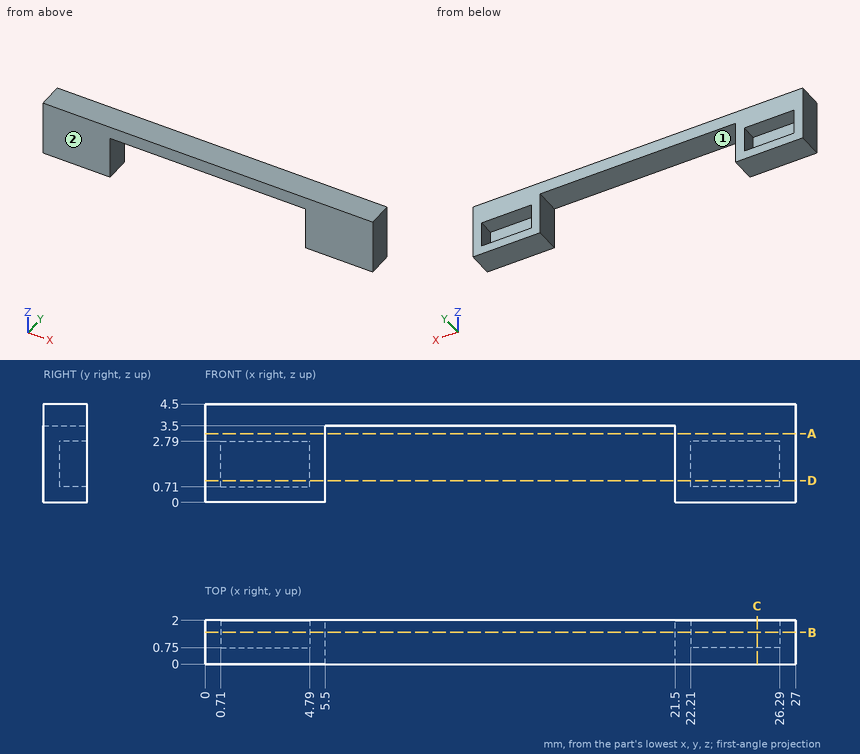
Verification items for this drawing (mm, ordinates from the low corner). Round coordinates to 2 decimals unless told otherwise and drop trailing zeros. Order: outer loops, then holes, each group sorted by start corner. A loop starts at its lowest first (then second) coordinate and runs counter-clockwise, first axis right, second up. Notation, with made-up numbers: M 44,9.5 L 61,9.5 A29 cw 61,46.5 Z; hole C 21,10.25 d10. An arc over 180 degrees is marked long. Answer in a Markdown table with one row per item. Add a question column.
Item 1: Sectioned sample at B-B, the plane y = 1.45. Enter the section's corners in (x, z).
Item 2: Sectioned sample at A-A, the plane z = 3.15. Enter the section's corners in (x, y).
Item 3: Sectioned sample at D-D, the plane z = 1. Enter the section's corners in (x, y), plus the area to 3 significant figures.
Item 4: Material ranges on L1, parallel to X at y = 1.45, z = 1.8; L2, parallel to X at y = 0.1, z = 2.3; L3, parallel to Z at x = 24, y = 1.2, recorded low to high. Write a range as [from, to].
Item 5: Sectioned sample at C-C, the plane x = 25.25. Enter the section's corners in (y, z), plus the area to 3 significant figures.
Item 6: Depth check by flat-ended pin: pin 1 Ø1.7 at (x, z) = (24.5, 2) entering from +Y. Enter the tip coordinate at first touch or a pass-through.
Item 7: Draft check along X on the marked faces 1 and 2. Enter one of: released by +X, released by -X, zero draft, split by the parting line, or undercut.
Filled in:
| question | item | result |
|---|---|---|
| 1 | outline | M 0,0 L 5.5,0 L 5.5,3.5 L 21.5,3.5 L 21.5,0 L 27,0 L 27,4.5 L 0,4.5 Z; hole M 0.71,0.71 L 4.79,0.71 L 4.79,2.79 L 0.71,2.79 Z; hole M 22.21,0.71 L 26.29,0.71 L 26.29,2.79 L 22.21,2.79 Z |
| 2 | outline | M 0,0 L 5.5,0 L 5.5,2 L 0,2 Z; M 21.5,0 L 27,0 L 27,2 L 21.5,2 Z |
| 3 | outline | M 0,0 L 5.5,0 L 5.5,2 L 4.79,2 L 4.79,0.75 L 0.71,0.75 L 0.71,2 L 0,2 Z; M 21.5,0 L 27,0 L 27,2 L 26.29,2 L 26.29,0.75 L 22.21,0.75 L 22.21,2 L 21.5,2 Z |
| 3 | area | 11.8 mm² |
| 4 | L1 | x = [0, 0.71], [4.79, 5.5], [21.5, 22.21], [26.29, 27] |
| 4 | L2 | x = [0, 5.5], [21.5, 27] |
| 4 | L3 | z = [0, 0.71], [2.79, 4.5] |
| 5 | outline | M 0,0 L 2,0 L 2,0.71 L 0.75,0.71 L 0.75,2.79 L 2,2.79 L 2,4.5 L 0,4.5 Z |
| 5 | area | 6.40 mm² |
| 6 | pin 1 | stops at y = 2 |
| 7 | face 1 | undercut |
| 7 | face 2 | zero draft |
